Work out the finished part from the listing and answer in its coordinate system (mm). A direction names the side the tool comes from. Coordinates: 2 decimals unless noted, no trailing zeros. Order: outer loops, then holes, each group sorted by start corner. A loop starts at its lowest first (then second) coordinate and runs counter-clockwise, first axis right, second up.
1. The part is cut by section A-A, the plane x = 34. Give the vertices of the cut face in (y, z), then the cut area to 3 significant figures.
2. A tool of negligible diameter and unlimited length cuts with its end or side. For faces 1 (the flat face through (-1, -143, -5)), 2 (the flat face through (90, -140, -5)), 3 (the flat face through (90, -143, -10)), 4 (the flat face through (-41, -142, -5)), 5 (the flat face through (28, -33, 3.5)), from which of +Z, -Z, +X, -X, +Y, -Y can it reach the whole face along a straight path? Write none if from no direction.
3. Determine the mould class of faces 6 (the flat face through (110, -143, -5)), 7 (the flat face through (-21, -143, -10)), 8 (the flat face through (70, -142, -5)) for opening direction X: +X half, -X half, draft (parallel to the pull), parting line (faces both ways), or undercut.
4. Find the intervals of material crossed by probe 1 along Y at (x, z) = (-77.5, 2.35); probe 2 along X at (y, z) = (72.5, 2.55); probe 3 along Z at (x, y) = (-33, -143), in increasing order.
5. The part is cut by section B-B, the plane y = 43. Give the vertices of the cut face in (x, z), then the cut area to 3 significant figures.
6. Flat-ended cylindrical pins translate along their axes: pin 1 Ø5.5 at (y, z) = (-142, -4.5) entering from +X; pin 2 Ø1.8 at (x, y) = (137.5, -142.5) entering from -Z; pin 3 Ø5 at (x, z) = (-28.5, -7) entering from +Y; pin 4 Ø5 at (x, y) = (-77.5, 72.5) entering from +Z. Find the tip coordinate at first contact, or state that the pin passes through.
Autodesk Fusion 360 part; units mm, degrees
sketch "Sketch1" plane through (0, 0, 0) normal (0, 0, 1) x (1, 0, 0)
  line L0 (-80, 75) -> (140, 75)
  line L1 (140, 75) -> (140, -145)
  line L2 (140, -145) -> (-80, -145)
  line L3 (-80, -145) -> (-80, 75)
  circle A0 centre (-77.5, 72.5) radius 1.5
  circle A1 centre (137.5, 72.5) radius 1.5
  circle A2 centre (137.5, -142.5) radius 1.5
  circle A3 centre (-77.5, -142.5) radius 1.5
  dimension "d1" = 220
  dimension "d2" = 220
  dimension "d3" = 3
  dimension "d4" = 3
  dimension "d5" = 3
  dimension "d6" = 3
  dimension "d7" = 2.5
  dimension "d8" = 2.5
  dimension "d9" = 2.5
  dimension "d10" = 2.5
  dimension "d11" = 2.5
  dimension "d12" = 2.5
  dimension "d13" = 2.5
  dimension "d14" = 2.5
extrude "Extrude1" add sketch "Sketch1" along normal blind 3.5
sketch "Sketch2" plane through (0, 0, 0) normal (0, 0, -1) x (1, 0, 0)
  circle A0 centre (137.5, 142.5) radius 1.5
  circle A1 centre (137.5, -72.5) radius 1.5
  circle A2 centre (-77.5, -72.5) radius 1.5
  circle A3 centre (-77.5, 142.5) radius 1.5
  line L0 (140, 145) -> (-80, 145)
  line L1 (-80, 145) -> (-80, -75)
  line L2 (-80, -75) -> (140, -75)
  line L3 (140, -75) -> (140, 145)
  line L4 (-41, 145) -> (-1, 145)
  line L5 (-1, 145) -> (-1, 140)
  line L6 (-1, 140) -> (-41, 140)
  line L7 (-41, 140) -> (-41, 145)
  line L8 (70, 145) -> (110, 145)
  line L9 (110, 145) -> (110, 140)
  line L10 (110, 140) -> (70, 140)
  line L11 (70, 140) -> (70, 145)
  dimension "d17" = 5
  dimension "d18" = 5
  dimension "d19" = 40
  dimension "d20" = 40
  dimension "d21" = 30
  dimension "d22" = 39
extrude "Extrude2" add sketch "Sketch2" along normal blind 10 contours L0 L8 L9 L10 L11 | L0 L4 L5 L6 L7
sketch "Sketch3" plane through (0, -145, 0) normal (0, -1, 0) x (1, 0, 0)
  line L0 (110, 0) -> (140, 0)
  line L1 (140, 0) -> (140, 3.5)
  line L2 (140, 3.5) -> (-80, 3.5)
  line L3 (-80, 3.5) -> (-80, 0)
  line L4 (-80, 0) -> (-41, 0)
  line L5 (-41, 0) -> (-41, -10)
  line L6 (-41, -10) -> (-1, -10)
  line L7 (-1, -10) -> (-1, 0)
  line L8 (-1, 0) -> (70, 0)
  line L9 (70, 0) -> (70, -10)
  line L10 (70, -10) -> (110, -10)
  line L11 (110, -10) -> (110, 0)
  circle A0 centre (-33, -5) radius 1.5
  circle A1 centre (-9, -5) radius 1.5
  circle A2 centre (78, -5) radius 1.5
  circle A3 centre (102, -5) radius 1.5
  dimension "d25" = 3
  dimension "d26" = 3
  dimension "d27" = 3
  dimension "d28" = 3
  dimension "d29" = 5
  dimension "d30" = 5
  dimension "d31" = 8
  dimension "d32" = 8
  dimension "d33" = 5
  dimension "d34" = 8
  dimension "d35" = 8
  dimension "d36" = 5
extrude "Extrude3" cut sketch "Sketch3" against normal blind 5 contours A0 | A1 | A2 | A3
Geometry says:
1. outline: (-145, 0) - (75, 0) - (75, 3.5) - (-145, 3.5) - close
1. area: 770 mm2
2. face 1: -Z, +Y, -Y
2. face 2: -Z, +X, -X, +Y
2. face 3: -Z, +X, -X, +Y, -Y
2. face 4: -Z, -X, +Y, -Y
2. face 5: +Z, +X, -X, +Y, -Y
3. face 6: +X half
3. face 7: draft
3. face 8: undercut
4. probe 1: y = -145 to -144, -141 to 71, 74 to 75
4. probe 2: x = -80 to -79, -76 to 136, 139 to 140
4. probe 3: z = -10 to -6.5, -3.5 to 3.5
5. outline: (-80, 0) - (140, 0) - (140, 3.5) - (-80, 3.5) - close
5. area: 770 mm2
6. pin 1: stops at x = 110
6. pin 2: passes through
6. pin 3: stops at y = -140
6. pin 4: stops at z = 3.5
